Geometry check sheet. Reference: the model listing, model coordinates, mm. A direction names the side the tool comes from. Give positions to 0.01 mm unless a question says otherwise; leave off trailing zeros. Loops run counter-clockwise (first coordinate to the right, second up) from the corner with the lowest first, then second, coordinate; pieces in that order, holes last.
1. Cross-section at A-A, the plane z = 0. Record the cut outline in (x, y).
2. Tool access check on faces 1 (the flat face through (2, 0, 6.045)), 2 (the flat face through (-2, 2, 3.48)), 3 (the flat face through (0.8, 1.37, 5.41)). Record the directions out of +Z, -Z, +X, -X, +Y, -Y that give a thin tool (end or side, any length) a straight path to the whole face; none if there is none.
3. Cross-section at C-C, the plane y = -3. Record the cut outline in (x, z), plus the area to 3 significant figures.
4. Cross-section at B-B, the plane z = 4.5. Record the cut outline in (x, y).
5. Material ranges on L1, parallel to Z at x = -3, y = 2.75; L2, parallel to Z at x = 2.75, y = -1.5; L3, parallel to Y at x = 3.25, z = 5, recorded low to high.
6. Go/stop test with flat-tipped pins: pin 1 Ø0.5 at (x, y) = (0, -1.5) entering from +Z; pin 2 Ø0.6 at (x, y) = (-1, 0.5) entering from +Z; pin 3 Ø0.6 at (x, y) = (1, -1) entering from +Z; pin 4 Ø4.5 at (x, y) = (-1.5, -2) entering from -Z. Record where each tip stops, or that it passes through.
7. Cross-section at D-D, the plane y = 4. Record the cut outline in (x, z).
8. Release check for a two-part mould opening along X. For faces 4 (the cylindrical face through (-2.79, -3.64, 3.66)), 5 (the flat face through (1.588, 0, 5.4)), 6 (the flat face through (0, 0, -6.045)) record: +X half, -X half, draft (parallel to the pull), parting line (faces both ways), or undercut.
from build123d import *

# Parameters (mm, degrees)
CUT_EXTRUDE1_START = 5.01904
CUT_EXTRUDE1_DEPTH = 2.02616
SKETCH4_R          = 1.833087105
CUT_EXTRUDE2_DEPTH = 1.02616
CUT_EXTRUDE2_DRAFT = -45


with BuildPart() as part:
    # Sketch2 → Revolve1 (revolve)
    with BuildSketch(Plane(origin=(0, 0, 0), x_dir=(0, 0, -1), z_dir=(1, 0, 0))):
        with BuildLine():
            Line((-6.0452, 1.5875), (-6.0452, 2.2225))
            ThreePointArc((-6.0452, 2.2225), (-5.130252118, 3.57733025), (-3.842657143, 4.5847))
            Line((-3.842657143, 4.5847), (-3.4798, 4.5847))
            Line((-3.4798, 4.5847), (-3.4798, 2.413))
            Line((-3.4798, 2.413), (5.25145, 2.413))
            Line((5.25145, 2.413), (6.0452, 1.61925))
            Line((6.0452, 1.61925), (6.0452, 0))
            Line((6.0452, 0), (-4.102496448, 0))
            Line((-4.102496448, 0), (-5.01904, 1.5875))
            Line((-5.01904, 1.5875), (-6.0452, 1.5875))
        make_face()
    revolve(axis=Axis((0, 0, 6.0452), (0, 0, -1)))

    # Sketch3 → Cut-Extrude1 (cut, through all)
    with BuildSketch(Plane.XY.offset(CUT_EXTRUDE1_START)):
        Polygon((0, 1.833087105), (-1.5875, 0.916543552), (-1.5875, -0.916543552), (0, -1.833087105), (1.5875, -0.916543552), (1.5875, 0.916543552), align=None)
    extrude(amount=CUT_EXTRUDE1_DEPTH, mode=Mode.SUBTRACT)


with BuildPart() as cut_extrude2_tool:
    # Sketch4 → Cut-Extrude2 (with draft: the straight prism first)
    with BuildSketch(Plane.XY.offset(6.0452)):
        Circle(SKETCH4_R)
    extrude(amount=-CUT_EXTRUDE2_DEPTH)
    # Cut-Extrude2: the draft: its side faces are tilted about the plane it starts from
    cut_extrude2_sides = [cut_extrude2_tool.faces().sort_by_distance(p)[0] for p in [
        (-1.833087105, 0, 5.53212),
    ]]
    draft(cut_extrude2_sides, Plane.XY.offset(6.0452), CUT_EXTRUDE2_DRAFT)


with BuildPart() as part_1:
    add(part.part)

    # Cut-Extrude2: cut by cut_extrude2_tool
    add(cut_extrude2_tool.part, mode=Mode.SUBTRACT)


solid = part_1.part
Result:
1. outline: circle Ø4.83 at (0, 0)
2. face 1: +Z, +X, -X, +Y, -Y
2. face 2: -Z
2. face 3: +Z
3. outline: (-3.47, 3.48) - (3.47, 3.48) - (3.47, 3.84) arc R4.3 ccw to (-3.47, 3.84) - close
3. area: 11.0 mm2
4. outline: circle Ø8.3 at (0, 0); hole circle Ø1.38 at (0, 0)
5. L1: z = 3.48 to 4.6
5. L2: z = 3.48 to 5.5
5. L3: y = -1.79 to 1.79
6. pin 1: stops at z = 5.02
6. pin 2: stops at z = 4.92
6. pin 3: stops at z = 5.93
6. pin 4: stops at z = -6.05
7. outline: (-2.24, 3.48) - (2.24, 3.48) - (2.24, 3.84) arc R3.39 ccw to (-2.24, 3.84) - close
8. face 4: parting line
8. face 5: undercut
8. face 6: draft
